Part model, mm, in its own coordinate system. Give positions to 0.01 mm unless a question says otherwise; leave off trailing zeros. Write each loop counter-clockwise with the first axis right and the second up, starting at its lowest first coordinate (ties: lowest second). Pieces come first, ordered by that corner, then holes. Notation, with made-up numbers: M 85.25,17 L 134.25,17 A21 cw 134.25,31 Z; hole C 89.5,14.5 d11. An arc over 180 degrees is marked long. Use a Markdown table: item, result.
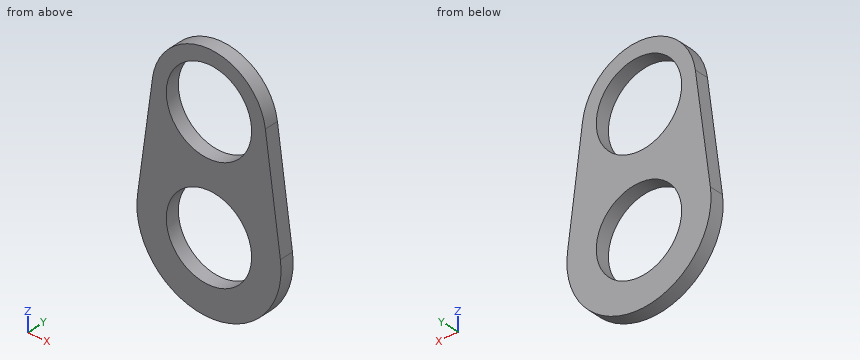
Autodesk Inventor part; units mm, degrees
ref_plane "YZ Plane" through (0, 0, 0) normal (1, 0, 0) x (0, 1, 0)
ref_plane "XZ Plane" through (0, 0, 0) normal (0, 1, 0) x (-1, 0, 0)
ref_plane "XY Plane" through (0, 0, 0) normal (0, 0, 1) x (1, 0, 0)
sketch "Sketch1" plane through (0, 0, 0) normal (0, 1, 0) x (-1, 0, 0)
  circle A0 centre (0, 0) radius 15.24 construction
  circle A1 centre (0, 0) radius 16.51 construction
  circle A2 centre (0, -38.1) radius 22.86 construction
  circle A3 centre (0, -38.1) radius 24.13 construction
  circle A4 centre (0, 0) radius 14.2875
  circle A5 centre (0, -38.1) radius 14.2875
  circle A6 centre (0, 0) radius 19.05 construction
  circle A7 centre (0, -38.1) radius 24.13 construction
  line L0 (18.8799, 2.54) -> (23.9145, -34.8827)
  line L1 (-18.8799, 2.54) -> (-23.9145, -34.8827)
  arc A8 (18.8799, 2.54) -> (-18.8799, 2.54) centre (0, 0) ccw
  arc A9 (-23.9145, -34.8827) -> (23.9145, -34.8827) centre (0, -38.1) ccw
  dimension "d0" = 30.48
  dimension "d2" = 1.27
  dimension "d3" = 45.72
  dimension "d5" = 1.27
  dimension "d6" = 28.575
  dimension "d7" = 4.7625
  dimension "d8" = 1.27
extrude "Extrusion1" add sketch "Sketch1" along normal blind 4.7625
properties part number "Train_006_Gearbox1"
1. Cut at A-A, the plane x = 0. Give the cut face in (y, z).
Findings below:
| item | result |
|---|---|
| outline | M 0,-62.23 L 4.76,-62.23 L 4.76,-52.39 L 0,-52.39 Z; M 0,-23.81 L 4.76,-23.81 L 4.76,-14.29 L 0,-14.29 Z; M 0,14.29 L 4.76,14.29 L 4.76,19.05 L 0,19.05 Z |
2. Cut at B-B, the plane z = -38.1. Give the cut face in (x, y), then the cut area to 3 significant figures.
Findings below:
| item | result |
|---|---|
| outline | M -24.13,0 L -14.29,0 L -14.29,4.76 L -24.13,4.76 Z; M 14.29,0 L 24.13,0 L 24.13,4.76 L 14.29,4.76 Z |
| area | 93.7 mm2 |
3. Cut at C-C, the plane y = 1.4. State how many separate pieces and enclosed holes the cut face has, then the cut area to 3 significant figures.
Findings below:
| item | result |
|---|---|
| separate pieces | 1 |
| enclosed holes | 2 |
| area | 1,860 mm2 |
4. Drop flat-ended pins along their axis: P1, Ø2, axis at x = -17.5, y = 1.5, coming from the -Z side; P2, Ø1, axis at y = 2, z = -1, coming from the -X side. Give the stop position or say it passes through.
Findings below:
| item | result |
|---|---|
| P1 | z = -55.71 |
| P2 | x = -19.42 |
5. Cut at D-D, the plane x = 7.5. Give the cut face in (y, z).
Findings below:
| item | result |
|---|---|
| outline | M 0,-61.03 L 4.76,-61.03 L 4.76,-50.26 L 0,-50.26 Z; M 0,-25.94 L 4.76,-25.94 L 4.76,-12.16 L 0,-12.16 Z; M 0,12.16 L 4.76,12.16 L 4.76,17.51 L 0,17.51 Z |
6. Drill centre lines: L1, parallel to Z at x = 0, y = 1; L2, parallel to Z at x = -13, y = 1.7; L3, parallel to X at y = 4.45, z = -1.5. Where is each one in solid material? Low to high.
Findings below:
| item | result |
|---|---|
| L1 | -62.23 to -52.39, -23.81 to -14.29, 14.29 to 19.05 |
| L2 | -58.43 to -44.03, -32.17 to -5.93, 5.93 to 13.92 |
| L3 | -19.42 to -14.21, 14.21 to 19.42 |
